Geometry: final body of the model. Coordinates: model frame, mm. A direction names the side the tool comes from. Give positions to 0.01 mm unless a question says otherwise; leave off trailing zeros. Loops run counter-clockwise (first coordinate to the right, second up) from the corner with the lowest first, then second, coordinate; pieces in that order, holes last. Notation, with made-up numbers: (16.5, -15) -> (35.5, -15) arc R31 cw to (35.5, 16) -> close; hole circle Ø5 at (8, 50). An arc over 180 degrees is marked (long way). Answer in a Markdown table with one row per item. Add a question column.
1) Draft query along Y for faces 1 (the flat face through (7, -14, 394)), 2 (the flat face through (7, -15, 394)), 3 (the flat face through (0.7, -7.4, 0)). Return one class per face: +Y half, -Y half, draft (parallel to the pull), parting line (faces both ways), or undercut.
2) Line query: line 1 (Z direction, x = 14.55, y = -7.5); line 2 (Z direction, x = 14.75, y = -7); line 3 (Y direction, x = 0.55, z = 725). Output: solid intervals per line, ascending. Write a range as from..to.
3) Section query A-A (x = 11.5). Return the cut outline in (y, z), plus the area to 3 significant figures.
4) Section query B-B (z = 470). Return the cut outline in (x, y).
5) Access query for faces 4 (the flat face through (1, -8, 394)), 5 (the flat face through (0, -8, 394)). Directions: +Z, -Z, +X, -X, +Y, -Y. A direction counts if a zero-diameter tool reaches every point of the face in a straight line with its end or side. Return the directions, or none.
```python
from build123d import *

# Parameters (mm, degrees)
SKETCH_1_W          = 15
SKETCH_1_H          = 15
SKETCH_1_W_2        = 13
SKETCH_1_H_2        = 13
EXTRUDE_1_DEPTH     = 800
SKETCH_4_R          = 1.5
CUT_EXTRUDE_3_DEPTH = 801.281200579
SKETCH_5_R          = 1.65
CUT_EXTRUDE_4_DEPTH = 801.281200579


with BuildPart() as part:
    # 草图1 → 拉伸-薄壁1 (new body)
    with BuildSketch(Plane.XY):
        with Locations((7.5, -7.5)):
            Rectangle(SKETCH_1_W, SKETCH_1_H)
        with Locations((7.5, -7.5)):
            Rectangle(SKETCH_1_W_2, SKETCH_1_H_2, mode=Mode.SUBTRACT)
    extrude(amount=EXTRUDE_1_DEPTH)

    # 草图4 → 切除-拉伸3 (cut, through all)
    with BuildSketch(Plane(origin=(15, 0, 0), x_dir=(0, 0, -1), z_dir=(1, 0, 0))):
        with Locations(Location((-790, -7.5, 0), (0, 0, 90))):
            Circle(SKETCH_4_R)
    extrude(amount=-CUT_EXTRUDE_3_DEPTH, mode=Mode.SUBTRACT)

    # 草图5 → 切除-拉伸4 (cut, through all)
    with BuildSketch(Plane(origin=(15, 0, 0), x_dir=(0, 0, -1), z_dir=(1, 0, 0))):
        with Locations(Location((-280, -7.5, 0), (0, 0, 90))):
            Circle(SKETCH_5_R)
        with Locations(Location((-295, -7.5, 0), (0, 0, 90))):
            Circle(SKETCH_5_R)
        with Locations(Location((-725, -7.5, 0), (0, 0, 90))):
            Circle(SKETCH_5_R)
        with Locations(Location((-740, -7.5, 0), (0, 0, 90))):
            Circle(SKETCH_5_R)
    extrude(amount=-CUT_EXTRUDE_4_DEPTH, mode=Mode.SUBTRACT)


solid = part.part
```
Evaluation:
| question | item | result |
|---|---|---|
| 1 | face 1 | undercut |
| 1 | face 2 | -Y half |
| 1 | face 3 | draft |
| 2 | line 1 | 0..278.35, 281.65..293.35, 296.65..723.35, 726.65..738.35, 741.65..788.5, 791.5..800 |
| 2 | line 2 | 0..278.43, 281.57..293.43, 296.57..723.43, 726.57..738.43, 741.57..788.59, 791.41..800 |
| 2 | line 3 | -15..-9.15, -5.85..0 |
| 3 | outline | (-15, 0) -> (-14, 0) -> (-14, 800) -> (-15, 800) -> close; (-1, 0) -> (0, 0) -> (0, 800) -> (-1, 800) -> close |
| 3 | area | 1,600 mm² |
| 4 | outline | (0, -15) -> (15, -15) -> (15, 0) -> (0, 0) -> close; hole (1, -14) -> (14, -14) -> (14, -1) -> (1, -1) -> close |
| 5 | face 4 | +Z, -Z |
| 5 | face 5 | +Z, -Z, -X, +Y, -Y |
